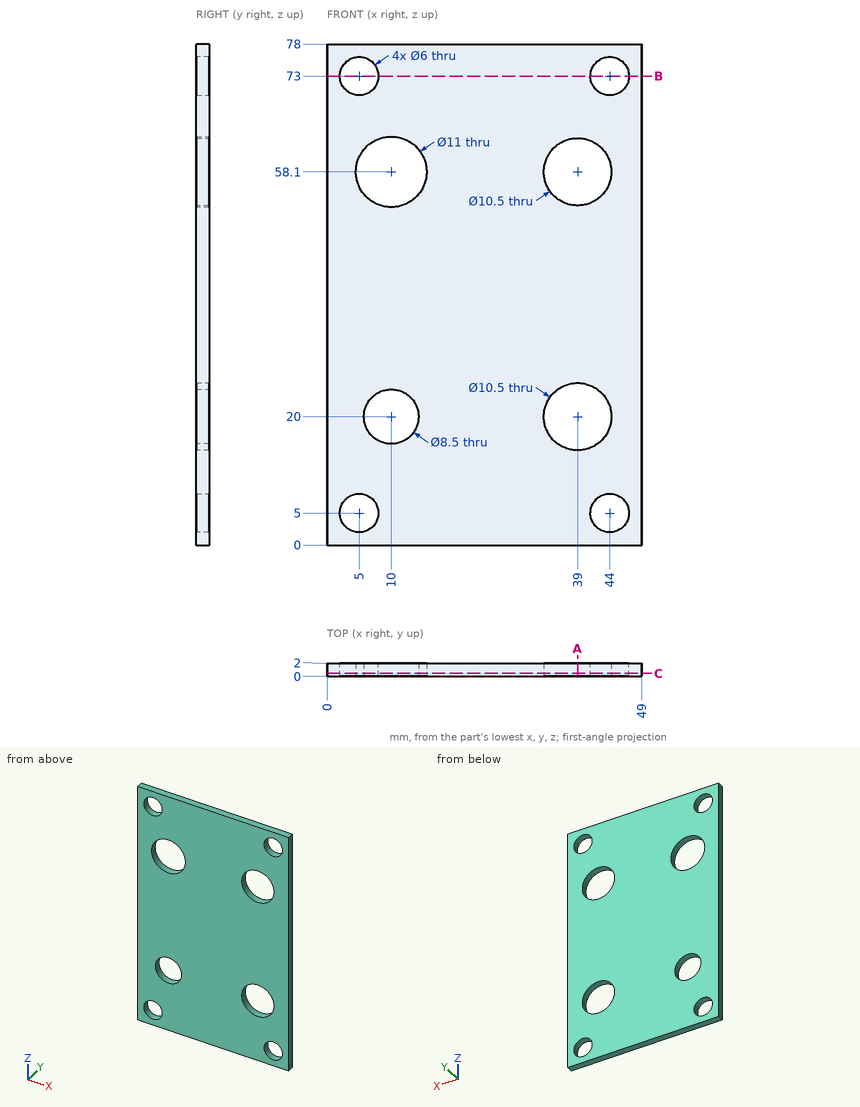
Print and shaded views of the part. All mm, measured from the part's lowest x, y and z. Round coordinates to 2 decimals unless told otherwise and drop trailing zeros. Write each loop counter-clockwise with the first axis right and the second up, starting at its lowest first coordinate (ties: lowest second). Pieces come first, ordered by that corner, then holes. Notation, with made-up numbers: (-7, -25) - (36, -25) arc R23 ccw to (36, -4) - close; hole circle Ø9 at (70.25, 12). An arc over 180 degrees is marked (long way). Use CSV: the item, a comma, the result in double quotes. Start each with the question number.
Item 1: Band-saw the part on C-C (y = 0.4). State how many separate pieces and enclosed holes the cut face has, and give its area (3 significant figures).
Item 2: Pin check, flat tip, straight feed: P1, Ø7.5, axis at x = 10, z = 20, coming from the -Y side. Stop position of the tip, or through.
Item 3: Drill centre lines: L1, parallel to X at y = 1.8, z = 58.5; L2, parallel to Z at x = 3.5, y = 1.2; L3, parallel to X at y = 1.4, z = 3. Where is each one in solid material? Low to high. Write a range as [from, to].
Item 4: Band-saw the part on B-B (z = 73). Write the cut outline in (x, y).
Item 5: Band-saw the part on A-A (x = 39). Write the cut outline in (y, z).
Checked values:
1,separate pieces,"1"
1,enclosed holes,"8"
1,area,"3,380 mm²"
2,P1,"passes through"
3,L1,"x = [0, 4.51], [15.49, 33.77], [44.23, 49]"
3,L2,"z = [0, 2.4], [7.6, 70.4], [75.6, 78]"
3,L3,"x = [0, 2.76], [7.24, 41.76], [46.24, 49]"
4,outline,"(0, 0) - (2, 0) - (2, 2) - (0, 2) - close; (8, 0) - (41, 0) - (41, 2) - (8, 2) - close; (47, 0) - (49, 0) - (49, 2) - (47, 2) - close"
5,outline,"(0, 0) - (2, 0) - (2, 14.75) - (0, 14.75) - close; (0, 25.25) - (2, 25.25) - (2, 52.85) - (0, 52.85) - close; (0, 63.35) - (2, 63.35) - (2, 78) - (0, 78) - close"
